Input: part model. Units: mm. Frame: model coordinates. Give positions to 0.01 mm unless a question says otherwise; leave off trailing zeros. Order: outer loops, then holes, each group sorted by start corner. A loop starts at its lowest first (then second) coordinate and runs counter-clockwise, first axis right, second up. Notation, with made-up numbers: M 58,25.5 L 68,25.5 A16 cw 68,33.5 Z; hole C 23.5,67.25 d1. An arc over 180 degrees is marked long. Use a Markdown table: item, result.
Autodesk Inventor part; units mm, degrees
ref_plane "YZ Plane" through (0, 0, 0) normal (1, 0, 0) x (0, 1, 0)
ref_plane "XZ Plane" through (0, 0, 0) normal (0, 1, 0) x (-1, 0, 0)
ref_plane "XY Plane" through (0, 0, 0) normal (0, 0, 1) x (1, 0, 0)
sketch "Sketch1" plane through (0, 0, 0) normal (0, 1, 0) x (-1, 0, 0)
  line L0 (-1.958, 8.8218) -> (-25.4378, 0.9475)
  line L1 (-26.3747, 3.741) -> (-2.8949, 11.6153)
  line L2 (-1.958, 8.8218) -> (-2.8949, 11.6153)
  line L3 (-25.4378, 0.9475) -> (-26.3747, 3.741)
  point P0 (0, 0)
  point P1 (-9.2456, 5.0352)
  dimension "d0" = 24.765
  dimension "d5" = 2.9464
extrude "Extrusion1" add sketch "Sketch1" along normal blind 48.895
fillet "Fillet1" radius 1.5875 1 edges at (26.3747, 24.4475, 3.741)
properties part number "Lidar Sensor Case Piece 4"
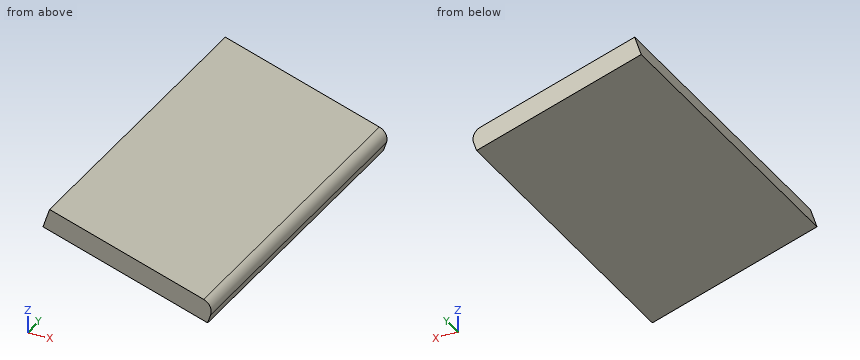
1) Cut plane C-C on x = 23.5. Return loops of the section in (y, z) (3 decimals), and give its area (3 significant figures).
Response values:
| item | result |
|---|---|
| outline | M 0,1.597 L 48.895,1.597 L 48.895,4.705 L 0,4.705 Z |
| area | 152 mm² |
2) First-contact query: pin 1 Ø2 at (x, y) = (21.5, 18) entering from -Z; pin 2 Ø1.5 at (x, y) = (21, 36) entering from +Z (3 decimals); pin 3 Ø8 at (x, y) = (23.5, 32) entering from +Z. Flat tips, straight axial feed; report the tip coordinate or a pass-through.
Response values:
| item | result |
|---|---|
| pin 1 | stops at z = 1.93 |
| pin 2 | stops at z = 5.795 |
| pin 3 | stops at z = 6.05 |
3) Cut plane B-B on z = 7.75. Return loops of the section in (x, y) (3 decimals).
Response values:
| item | result |
|---|---|
| outline | M 5.154,0 L 14.421,0 L 14.421,48.895 L 5.154,48.895 Z |
4) Cut plane A-A on y = 7. Return loops of the section in (x, z) (1 decimal).
Response values:
| item | result |
|---|---|
| outline | M 2,8.8 L 25.4,0.9 L 25.9,2.2 A1.6 ccw 24.9,4.2 L 2.9,11.6 Z |
5) Material intervals for line 1 (Z direction, x = 13, y = 27); line 2 (Z direction, x = 9.5, y = 44), sorted ascending. Write a range as from..to.
Response values:
| item | result |
|---|---|
| line 1 | z = 5.12..8.23 |
| line 2 | z = 6.29..9.4 |
